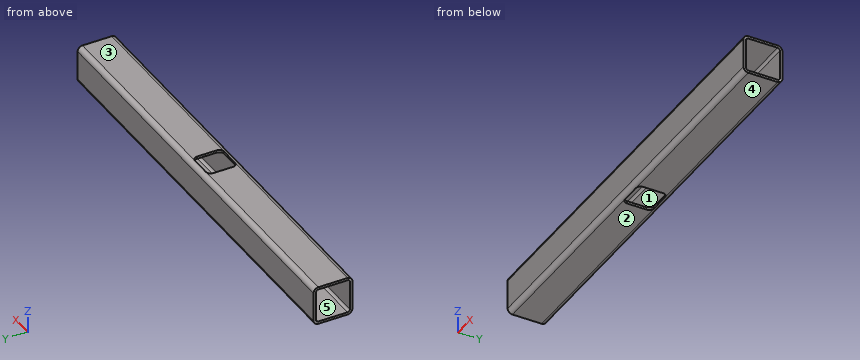
Autodesk Inventor part; units mm, degrees
ref_plane "YZ Plane" through (0, 0, 0) normal (1, 0, 0) x (0, 1, 0)
ref_plane "XZ Plane" through (0, 0, 0) normal (0, 1, 0) x (-1, 0, 0)
ref_plane "XY Plane" through (0, 0, 0) normal (0, 0, 1) x (1, 0, 0)
sketch "Sketch5" plane through (0, 0, 0) normal (1, 0, 0) x (0, 1, 0)
  line L0 (-38.1, 50.8) -> (38.1, 50.8)
  line L1 (50.8, 38.1) -> (50.8, -38.1)
  line L2 (38.1, -50.8) -> (-38.1, -50.8)
  line L3 (-50.8, -38.1) -> (-50.8, 38.1)
  line L4 (-50.8, 50.8) -> (50.8, -50.8) construction
  line L5 (50.8, 50.8) -> (-50.8, -50.8) construction
  arc A0 (50.8, 38.1) -> (38.1, 50.8) centre (38.1, 38.1) ccw
  arc A1 (38.1, -50.8) -> (50.8, -38.1) centre (38.1, -38.1) ccw
  arc A2 (-50.8, -38.1) -> (-38.1, -50.8) centre (-38.1, -38.1) ccw
  arc A3 (-38.1, 50.8) -> (-50.8, 38.1) centre (-38.1, 38.1) ccw
  line L6 (44.45, -38.1) -> (44.45, 38.1)
  arc A4 (44.45, 38.1) -> (38.1, 44.45) centre (38.1, 38.1) ccw
  line L7 (38.1, 44.45) -> (-38.1, 44.45)
  arc A5 (-38.1, 44.45) -> (-44.45, 38.1) centre (-38.1, 38.1) ccw
  line L8 (-44.45, 38.1) -> (-44.45, -38.1)
  arc A6 (-44.45, -38.1) -> (-38.1, -44.45) centre (-38.1, -38.1) ccw
  line L9 (-38.1, -44.45) -> (38.1, -44.45)
  arc A7 (38.1, -44.45) -> (44.45, -38.1) centre (38.1, -38.1) ccw
  point P0 (0, 0)
  dimension "d6" = 101.6
  dimension "d7" = 101.6
  dimension "d8" = 12.7
  dimension "d9" = 6.35
extrude "Extrusion4" add sketch "Sketch5" along normal mid plane 1111.25
sketch "Sketch6" plane through (-555.625, -38.1, 50.8) normal (0, 0, 1) x (1, 0, 0)
  line L0 (530.225, 0) -> (581.025, 0)
  line L1 (593.725, 12.7) -> (593.725, 63.5)
  line L2 (581.025, 76.2) -> (530.225, 76.2)
  line L3 (517.525, 63.5) -> (517.525, 12.7)
  line L4 (517.525, 0) -> (593.725, 76.2) construction
  line L5 (593.725, 0) -> (517.525, 76.2) construction
  arc A0 (530.225, 76.2) -> (517.525, 63.5) centre (530.225, 63.5) ccw
  arc A1 (593.725, 63.5) -> (581.025, 76.2) centre (581.025, 63.5) ccw
  arc A2 (517.525, 12.7) -> (530.225, 0) centre (530.225, 12.7) ccw
  arc A3 (581.025, 0) -> (593.725, 12.7) centre (581.025, 12.7) ccw
  point P0 (555.625, 38.1)
  dimension "d12" = 76.2
  dimension "d13" = 76.2
  dimension "d14" = 12.7
extrude "Extrusion5" cut sketch "Sketch6" against normal blind 177.8
properties part number "Model-2_Base Tube-1" material "SS304"
Can you work these out from the model? Positions are in its coordinate system, mm. Face numbers are marked on the shaded views. A direction names the side the tool comes from. Give positions to 0.01 mm unless a question says otherwise; leave off trailing zeros. Order: outer loops, then holes, each group sorted by start corner. A loop starts at its lowest first (then second) coordinate and runs counter-clockwise, first axis right, second up. Notation, with made-up numbers: M 14.5,-24 L 45.5,-24 A22 cw 45.5,-10 Z; hole C 75,-33 d1. An arc over 180 degrees is marked long. Use a Markdown table: item, result. Add a question column.
Item 1: We'd pull the mould along Z, two halves only. Please class the marked faces 1, 2 and 3: +Z half, -Z half, draft (parallel to the pull), parting line (faces both ways), or undercut.
Item 2: Will these pins go through, and if not, where does the flat tip stop? pin 1 (7 mm diameter, centred on x = 0.5, z = 48, fed in from +Y); pin 2 (1 mm diameter, centred on x = 167.5, z = 40.5, fed in from -Y); pin 3 (1.9 mm diameter, centred on x = -12.5, z = -49, fed in from -Y).
Item 3: Suppose I cut it at A-A (y = 11). List the corners of the cut face in (x, z) for me (3 decimals), then the cut area to 3 significant figures.
Item 4: Suppose I cut it at B-B (z = -15.5). List the corners of the cut face in (x, y) for me (3 decimals), then the cut area to 3 significant figures.
Item 5: For the marked faces 4 and 5, which set-ups out of +Z, -Z, +X, -X, +Y, -Y let a thin tool reach every point of the face, with its end or its side?
Item 6: If I drill on L1, parallel to Z at x = 69.5, y = -34.5; L2, parallel to Z at x = 269, y = -42, over which ranges is the centre line in solid material (lowest first)? Write a range as [from, to].
Item 7: Suppose I cut it at C-C (x = -365.5). List the corners of the cut face in (y, z) for me, then the cut area to 3 significant figures.
Answer sheet:
| question | item | result |
|---|---|---|
| 1 | face 1 | undercut |
| 1 | face 2 | -Z half |
| 1 | face 3 | +Z half |
| 2 | pin 1 | stops at y = 49.07 |
| 2 | pin 2 | stops at y = -50.66 |
| 2 | pin 3 | stops at y = -45.99 |
| 3 | outline | M -555.625,-50.8 L -38.1,-50.8 L -38.1,-44.45 L -555.625,-44.45 Z; M -555.625,44.45 L -38.1,44.45 L -38.1,50.8 L -555.625,50.8 Z; M 38.1,-50.8 L 555.625,-50.8 L 555.625,-44.45 L 38.1,-44.45 Z; M 38.1,44.45 L 555.625,44.45 L 555.625,50.8 L 38.1,50.8 Z |
| 3 | area | 13,100 mm² |
| 4 | outline | M -555.625,-50.8 L 555.625,-50.8 L 555.625,-44.45 L -555.625,-44.45 Z; M -555.625,44.45 L 555.625,44.45 L 555.625,50.8 L -555.625,50.8 Z |
| 4 | area | 14,100 mm² |
| 5 | face 4 | -Z, +X, -X, +Y, -Y |
| 5 | face 5 | +X, -X |
| 6 | L1 | z = [-50.8, -44.45], [44.45, 50.8] |
| 6 | L2 | z = [-50.19, -43.11], [43.11, 50.19] |
| 7 | outline | M -50.8,-38.1 A12.7 ccw -38.1,-50.8 L 38.1,-50.8 A12.7 ccw 50.8,-38.1 L 50.8,38.1 A12.7 ccw 38.1,50.8 L -38.1,50.8 A12.7 ccw -50.8,38.1 Z; hole M -44.45,-38.1 A6.35 ccw -38.1,-44.45 L 38.1,-44.45 A6.35 ccw 44.45,-38.1 L 44.45,38.1 A6.35 ccw 38.1,44.45 L -38.1,44.45 A6.35 ccw -44.45,38.1 Z |
| 7 | area | 2,320 mm² |
